Design review of the part built by this model. Coordinates are the model's own, in mm. A direction names the side the tool comes from. Coordinates: 2 decimals unless noted, no trailing zeros. Order: outer loops, then holes, each group sorted by start corner. A loop starts at its lowest first (then second) coordinate and runs counter-clockwise, first axis right, second up. Notation, with made-up numbers: M 56.25,78.5 L 90.25,78.5 A27 ccw 90.25,107.5 Z; hole C 84.25,77 d11. An arc over 180 degrees is marked long. Answer as a JSON object with one key per item and string values.
from build123d import *

# Parameters (mm, degrees)
EXTRUDE1_DEPTH          = 2.6924
SKETCH2_OUTSIDE_W       = 34.708
SKETCH2_OUTSIDE_H       = 35.936
SKETCH2_OUTSIDE_R       = 3.96875
CUT_EXTRUDE1_DEPTH      = 6.3848
CUT_EXTRUDE1_TAPER      = 60
SKETCH17_R              = 5.1943
EXTRUDE3_DEPTH          = 0.7874
F_1_4_28_TAPPED_HOLE1_D = 5.4102


with BuildPart() as part:
    # Sketch1 → Extrude1 (new body, symmetric)
    with BuildSketch(Plane.XY):
        Polygon((3.96875, -2.291358881), (3.96875, 2.291358881), (0, 4.582717762), (-3.96875, 2.291358881), (-3.96875, -2.291358881), (0, -4.582717762), align=None)
    extrude(amount=EXTRUDE1_DEPTH, both=True)

    # Sketch2 outside → Cut-Extrude1 (cut, through all)
    with BuildSketch(Plane.XY.offset(2.6924)):
        Rectangle(SKETCH2_OUTSIDE_W, SKETCH2_OUTSIDE_H)
        Circle(SKETCH2_OUTSIDE_R, mode=Mode.SUBTRACT)
    extrude(amount=-CUT_EXTRUDE1_DEPTH, taper=CUT_EXTRUDE1_TAPER, mode=Mode.SUBTRACT)

    # Sketch17 → Extrude3 (add)
    with BuildSketch(Plane(origin=(0, 0, -2.6924), x_dir=(-1, 0, 0), z_dir=(0, 0, -1))):
        Circle(SKETCH17_R)
    extrude(amount=-EXTRUDE3_DEPTH)

    # 1/4-28 Tapped Hole1 (through all)
    with Locations(Plane.XY.offset(2.6924)):
        with Locations((0, 0)):
            Hole(F_1_4_28_TAPPED_HOLE1_D / 2)


solid = part.part
1) Add section A-A (z = -0.15). State the section outline as (x, y) points, and give its area (3 significant figures).
Taken from the geometry:
{"outline": "M -3.97,-2.29 L 0,-4.58 L 3.97,-2.29 L 3.97,2.29 L 0,4.58 L -3.97,2.29 Z; hole C 0,0 d5.41", "area": "31.6 mm2"}
2) Mouldability with a two-part tool opening along X and no side actions: class faces 5 (the cylindrical face through (5.19, 0.23, -2.3)), 6 (the cylindrical face through (-2.58, 0.81, -0.04)), 7 (the flat face through (-2.2, -2.2, -2.692)) as released by +X, released by -X, zero draft, split by the parting line, or undercut.
Taken from the geometry:
{"face 5": "split by the parting line", "face 6": "undercut", "face 7": "zero draft"}
3) Tool access review of faces 1 (the flat face through (2.01, 3.42, 0.43)), 2 (the flat face through (3.969, 0, 0)), 3 (the flat face through (-1.96, 3.45, 0.43)), 4 (the flat face through (-3.969, 0, 0)): name each direction out of +Z, -Z, +X, -X, +Y, -Y from which nothing blocks a thin tool from reaching the whole face with its end or side.
Taken from the geometry:
{"face 1": "+Z, +X, +Y", "face 2": "+Z, +X, +Y, -Y", "face 3": "+Z, -X, +Y", "face 4": "+Z, -X, +Y, -Y"}
4) Insertion check: pin 1 Ø1.5 at (y, z) = (0, 1.5) entering from +X; pin 2 Ø1 at (x, z) = (2, -0.5) entering from -Y. Each pin has a flat end and moves straight along its axis. Give the tip position at first contact, or say it passes through.
Taken from the geometry:
{"pin 1": "stops at x = 3.97", "pin 2": "stops at y = -3.72"}
5) To check wall thickness, follow L1, parallel to Y at x = 3.25, z = 0.05; L2, parallel to Z at x = -3.75, y = 2.5 (3 decimals); L3, parallel to Y at x = 1.5, z = -0.3. State the ranges of each line that lie inside material, in increasing order.
Taken from the geometry:
{"L1": "y = -2.71 to 2.71", "L2": "z = -2.692 to -1.905", "L3": "y = -3.72 to -2.25, 2.25 to 3.72"}
